Autodesk Inventor part; units mm, degrees
ref_plane "YZ Plane" through (0, 0, 0) normal (1, 0, 0) x (0, 1, 0)
ref_plane "XZ Plane" through (0, 0, 0) normal (0, 1, 0) x (-1, 0, 0)
ref_plane "XY Plane" through (0, 0, 0) normal (0, 0, 1) x (1, 0, 0)
sketch "Sketch1" plane through (0, 0, 0) normal (0, 1, 0) x (-1, 0, 0)
  line L0 (-32.5, 28) -> (32.5, 28)
  line L1 (32.5, 28) -> (32.5, -28)
  line L2 (32.5, -28) -> (-32.5, -28)
  line L3 (-32.5, -28) -> (-32.5, 28)
  line L4 (-32.5, 28) -> (32.5, -28) construction
  line L5 (32.5, 28) -> (-32.5, -28) construction
  circle A0 centre (4.5, 0) radius 11.15
  line L6 (-11, 15.5) -> (20, 15.5) construction
  line L7 (20, 15.5) -> (20, -15.5) construction
  line L8 (20, -15.5) -> (-11, -15.5) construction
  line L9 (-11, -15.5) -> (-11, 15.5) construction
  line L10 (-11, 15.5) -> (20, -15.5) construction
  line L11 (20, 15.5) -> (-11, -15.5) construction
  circle A1 centre (20, 15.5) radius 2
  line L12 (-11, 15.5) -> (20, 15.5) construction
  line L13 (20, 15.5) -> (20, -15.5) construction
  line L14 (20, -15.5) -> (-11, -15.5) construction
  line L15 (-11, -15.5) -> (-11, 15.5) construction
  circle A2 centre (-11, 15.5) radius 2
  line L16 (-11, -15.5) -> (-11, 15.5) construction
  line L17 (-11, 15.5) -> (20, 15.5) construction
  line L18 (20, 15.5) -> (20, -15.5) construction
  line L19 (20, -15.5) -> (-11, -15.5) construction
  circle A3 centre (-11, -15.5) radius 2
  line L20 (20, -15.5) -> (-11, -15.5) construction
  line L21 (-11, -15.5) -> (-11, 15.5) construction
  line L22 (-11, 15.5) -> (20, 15.5) construction
  line L23 (20, 15.5) -> (20, -15.5) construction
  circle A4 centre (20, -15.5) radius 2
  circle A5 centre (28.1317, 23.6317) radius 2
  line L24 (28.1317, 23.6317) -> (20, 15.5) construction
  circle A6 centre (-19.1317, 23.6317) radius 2
  circle A7 centre (-19.1317, -23.6317) radius 2
  circle A8 centre (28.1317, -23.6317) radius 2
  circle A9 centre (-22.5, -12) radius 3.15
  line L25 (32.5, 0) -> (-32.5, 0) construction
  circle A10 centre (-22.5, 12) radius 3.15
  point P0 (0, 0)
  point P1 (0, 0)
  dimension "d0" = 56
  dimension "d1" = 65
  dimension "d2" = 28
  dimension "d3" = 22.3
  dimension "d4" = 31
  dimension "d5" = 31
  dimension "d8" = 360
  dimension "d10" = 4
  dimension "d11" = 11.5
  dimension "d12" = 4
  dimension "d15" = 360
  dimension "d17" = 16
  dimension "d18" = 10
  dimension "d19" = 6.3
extrude "Extrusion1" add sketch "Sketch1" along normal blind 8
sketch "Sketch2" plane through (0, 8, 0) normal (0, 1, 0) x (1, 0, 0)
  circle A0 centre (-4.5, 0) radius 11.15 construction
  line L0 (16.65, -21.15) -> (-25.65, -21.15)
  line L1 (-25.65, -21.15) -> (-25.65, 21.15)
  line L2 (-25.65, 21.15) -> (16.65, 21.15)
  line L3 (16.65, 21.15) -> (16.65, -21.15)
  line L4 (16.65, -21.15) -> (-25.65, 21.15) construction
  line L5 (-25.65, -21.15) -> (16.65, 21.15) construction
  point P0 (0, 0)
  dimension "d22" = 42.3
  dimension "d23" = 42.3
extrude "Extrusion2" cut sketch "Sketch2" against normal blind 1
sketch "Sketch3" plane through (0, 8, 0) normal (0, 1, 0) x (1, 0, 0)
  circle A0 centre (22.5, -12) radius 3.15 construction
  circle A1 centre (22.5, 12) radius 3.15 construction
  circle A2 centre (22.5, -12) radius 5
  circle A3 centre (22.5, 12) radius 5
  point P0 (0, 0)
  dimension "d26" = 10
  dimension "d27" = 10
extrude "Extrusion3" cut sketch "Sketch3" against normal blind 5
sketch "Sketch4" plane through (0, 0, 0) normal (0, -1, 0) x (1, 0, 0)
  line L0 (32.5, -28) -> (-32.5, -28)
  line L1 (32.5, 28) -> (32.5, -28)
  line L2 (-32.5, 28) -> (32.5, 28)
  line L3 (-32.5, -28) -> (-32.5, 28)
  circle A0 centre (22.5, 12) radius 3.15
  circle A1 centre (-28.1317, -23.6317) radius 2
  circle A2 centre (-4.5, 0) radius 11.15
  circle A3 centre (-20, 15.5) radius 2
  circle A4 centre (11, 15.5) radius 2
  circle A5 centre (11, -15.5) radius 2
  circle A6 centre (-20, -15.5) radius 2
  circle A7 centre (-28.1317, 23.6317) radius 2
  circle A8 centre (19.1317, 23.6317) radius 2
  circle A9 centre (19.1317, -23.6317) radius 2
  circle A10 centre (22.5, -12) radius 3.15
  circle A11 centre (-20, 15.5) radius 3
  circle A12 centre (-20, -15.5) radius 3
  circle A13 centre (11, -15.5) radius 3
  circle A14 centre (11, 15.5) radius 3
  circle A15 centre (21, 18.5) radius 3
  line L4 (-32.5, -28) -> (-32.5, 28)
  line L5 (-32.5, 0) -> (32.5, 0) construction
  circle A16 centre (21, -18.5) radius 3
  point P0 (0, 0)
  dimension "d30" = 6
  dimension "d33" = 360
  dimension "d35" = 9.5
  dimension "d36" = 11.5
  dimension "d37" = 6
extrude "Extrusion4" cut sketch "Sketch4" against normal blind 5 contours A3 | A4 | A5 | A6 | A11 | A12 | A13 | A14 | A15 | A16
properties part number "Linear Rail Front Plate"
Geometry: final body of the model. Coordinates: model frame, mm. A direction names the side the tool comes from. Round coordinates to 2 decimals unless told otherwise and drop trailing zeros. Order: outer loops, then holes, each group sorted by start corner. A loop starts at its lowest first (then second) coordinate and runs counter-clockwise, first axis right, second up. Notation, with made-up numbers: (33.5, -22.5) - (51.5, -22.5) arc R26 ccw to (51.5, 4.5) - close; hole circle Ø2 at (33.5, 7.5). An arc over 180 degrees is marked (long way). Use CSV: the item, a comma, the result in double quotes. Start each with the question number.
Q1. Section query B-B (z = 0). Return loops of the section in (x, y).
Q2. Section query C-C (x = -4.5). Return loops of the section in (y, z).
Q3. Mould query, pull axis X, two halves, no side actions, for faces 4 (the face through (32.5, 4, 0)), 5 (the face through (11, 5, -13)), 6 (the face through (-32.5, 4, 0)). Classes: +X half, -X half, draft (parallel to the pull), parting line (faces both ways), or undercut.
Q4. Section query D-D (y = 2). State how many separate pieces and enclosed holes the cut face has, and give its area (3 significant figures).
Q5. Section query A-A (x = 11). Return loops of the section in (y, z), and give its area (3 significant figures).
Q6. Material intervals for line 1 along Z through (x, y) = (11, 3.3); line 2 along Z through (x, y) = (-5, 4.5); line 3 along X through (y, z) = (2.75, -12), sorted ascending. Write a range as from..to.
Q7. First-contact query: pin 1 (5 mm diameter, centred on x = 23.5, z = 14, fed in from +Y); pin 2 (6.5 mm diameter, centred on x = -20, z = -15.5, fed in from +Y); pin 3 (3 mm diameter, centred on x = 22, z = 19.5, fed in from -Y). Flat tips, straight axial feed; report the tip coordinate or a pass-through.
Q8. Access query for faces 1 (the face through (5, 7, 9)), 2 (the face through (-20.65, 2.46, -18.43)), 3 (the face through (-30.04, 3.94, 23.03)). Directions: +Z, -Z, +X, -X, +Y, -Y. A direction counts if a zero-diameter tool reaches every point of the face in a straight line with its end or side. Return the directions, or none.
Result set:
1,outline,"(-32.5, 0) - (-15.65, 0) - (-15.65, 7) - (-25.65, 7) - (-25.65, 8) - (-32.5, 8) - close; (6.65, 0) - (32.5, 0) - (32.5, 8) - (16.65, 8) - (16.65, 7) - (6.65, 7) - close"
2,outline,"(0, -28) - (8, -28) - (8, -21.15) - (7, -21.15) - (7, -11.15) - (0, -11.15) - close; (0, 11.15) - (7, 11.15) - (7, 21.15) - (8, 21.15) - (8, 28) - (0, 28) - close"
3,face 4,"+X half"
3,face 5,"undercut"
3,face 6,"-X half"
4,separate pieces,"1"
4,enclosed holes,"13"
4,area,"2,970 mm2"
5,outline,"(0, -28) - (8, -28) - (8, -21.15) - (7, -21.15) - (7, -17.5) - (5, -17.5) - (5, -18.5) - (0, -18.5) - close; (0, -12.5) - (5, -12.5) - (5, -13.5) - (7, -13.5) - (7, 13.5) - (5, 13.5) - (5, 12.5) - (0, 12.5) - close; (0, 18.5) - (5, 18.5) - (5, 17.5) - (7, 17.5) - (7, 21.15) - (8, 21.15) - (8, 28) - (0, 28) - close"
5,area,"330 mm2"
6,line 1,"z = -28..-18.5, -12.5..12.5, 18.5..28"
6,line 2,"z = -28..-11.14, 11.14..28"
6,line 3,"x = -32.5..19.35, 25.65..32.5"
7,pin 1,"stops at y = 3"
7,pin 2,"stops at y = 7"
7,pin 3,"stops at y = 5"
8,face 1,"+Y"
8,face 2,"-Y"
8,face 3,"+Y, -Y"
